The drawing under review shows one solid part. Ordinate dimensions are in mm from its lowest x, y, z. Coordinates: 2 decimals unless noted, no trailing zeros. Order: outer loops, then holes, each group sorted by start corner. A loop starts at its lowest first (then second) coordinate and runs counter-clockwise, first axis right, second up. Notation, with made-up numbers: (-10, -4) - (13, -4) arc R33 cw to (13, 28) - close; hole circle Ø7 at (-10.75, -18). An arc over 180 degrees is marked (long way). Answer in a Markdown table with one row per item.
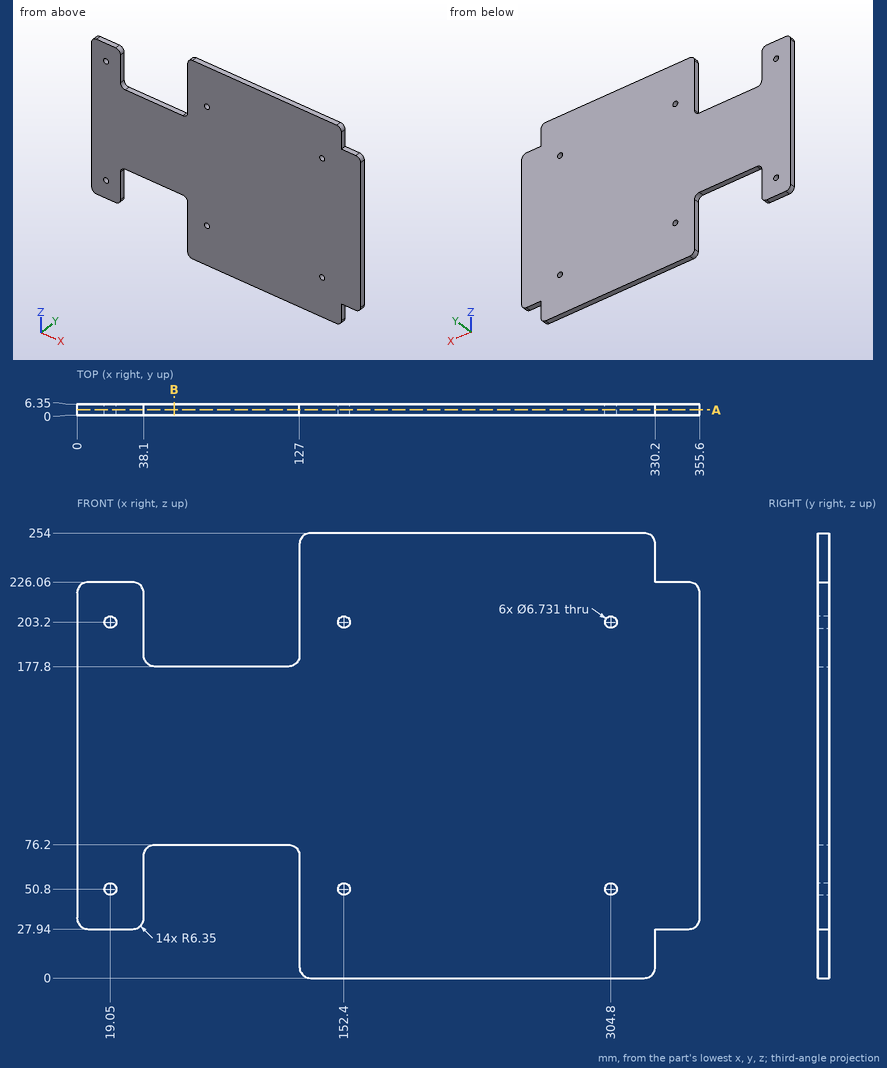
Item 1: To check wall thickness, follow line 1 (Z direction, x = 19.05, y = 1.5); line 2 (X direction, y = 2.75, z = 203.2); line 3 (Z direction, x = 304.8, y = 3). State the ranges of each line that lie inside material, in increasing order. Write a range as from..to.
Check values:
| item | result |
|---|---|
| line 1 | 27.94..47.43, 54.17..199.83, 206.57..226.06 |
| line 2 | 0..15.68, 22.42..38.1, 127..149.03, 155.77..301.43, 308.17..355.6 |
| line 3 | 0..47.43, 54.17..199.83, 206.57..254 |
Item 2: Clearance check with flat-ended pins moving along their axes: pin 1 Ø1.9 at (y, z) = (4.5, 19.5) entering from +X; pin 2 Ø6 at (x, z) = (304.8, 203.2) entering from -Y; pin 3 Ø3 at (x, y) = (65, 2) entering from -Z. State where each tip first meets the part, or that it passes through.
Check values:
| item | result |
|---|---|
| pin 1 | x = 330.2 |
| pin 2 | through |
| pin 3 | z = 76.2 |
Item 3: We need section B-B, the plane x = 55.5. Write out the cut boundary in (y, z), then the cut area to 3 significant figures.
Check values:
| item | result |
|---|---|
| outline | (0, 76.2) - (6.35, 76.2) - (6.35, 177.8) - (0, 177.8) - close |
| area | 645 mm^2 |
Item 4: We need section A-A, the plane y = 3. State how many separate pieces and enclosed holes the cut face has, then the cut area to 3 significant figures.
Check values:
| item | result |
|---|---|
| separate pieces | 1 |
| enclosed holes | 6 |
| area | 73,000 mm^2 |
